```python
from build123d import *

# Parameters (mm, degrees)
SKETCH1_R            = 60
SKETCH1_R_2          = 7.9
BOSS_EXTRUDE1_DEPTH  = 8
M6_CLEARANCE_HOLE1_D = 6.6
M3_CLEARANCE_HOLE1_D = 3.6
SKETCH8_R            = 4.2
CUT_EXTRUDE1_DEPTH   = 2.7
CHAMFER1_SIZE        = 0.5


with BuildPart() as part:
    # Sketch1 → Boss-Extrude1 (new body)
    with BuildSketch(Plane.XY):
        Circle(SKETCH1_R)
        Circle(SKETCH1_R_2, mode=Mode.SUBTRACT)
    extrude(amount=BOSS_EXTRUDE1_DEPTH)

    # M6 Clearance Hole1 (through all)
    with Locations(Plane.XY.offset(8)):
        with Locations((-37.123106012, 37.123106012), (0, 52.5), (37.123106012, 37.123106012), (52.5, 0), (37.123106012, -37.123106012), (0, -52.5), (-37.123106012, -37.123106012), (-52.5, 0)):
            Hole(M6_CLEARANCE_HOLE1_D / 2)

    # M3 Clearance Hole1 (through all)
    with Locations(Plane.XY.offset(8)):
        with Locations((0, 12.5), (0, -12.5), (0, 0)):
            Hole(M3_CLEARANCE_HOLE1_D / 2)

    # Sketch8 → Cut-Extrude1 (cut)
    with BuildSketch(Plane.XY.offset(8)):
        with Locations((30, 0)):
            Circle(SKETCH8_R)
        with Locations((26.56368077, -13.941695161)):
            Circle(SKETCH8_R)
        with Locations((17.041942402, -24.689515977)):
            Circle(SKETCH8_R)
        with Locations((3.616100408, -29.781266223)):
            Circle(SKETCH8_R)
        with Locations((-10.638146611, -28.050487281)):
            Circle(SKETCH8_R)
        with Locations((-22.455322445, -19.893679747)):
            Circle(SKETCH8_R)
        with Locations((-29.128254523, -7.179469929)):
            Circle(SKETCH8_R)
        with Locations((-29.128254523, 7.179469929)):
            Circle(SKETCH8_R)
        with Locations((-22.455322445, 19.893679747)):
            Circle(SKETCH8_R)
        with Locations((-10.638146611, 28.050487281)):
            Circle(SKETCH8_R)
        with Locations((3.616100408, 29.781266223)):
            Circle(SKETCH8_R)
        with Locations((17.041942402, 24.689515977)):
            Circle(SKETCH8_R)
        with Locations((26.56368077, 13.941695161)):
            Circle(SKETCH8_R)
    extrude(amount=-CUT_EXTRUDE1_DEPTH, mode=Mode.SUBTRACT)

    # Chamfer1
    chamfer1_edges = [part.edges().sort_by_distance(p)[0] for p in [
        (25.8, 0, 5.3),
        (25.8, 0, 8),
        (-33.823106012, 37.123106012, 8),
        (-33.823106012, 37.123106012, 0),
        (-60, 0, 0),
        (-49.2, 0, 8),
        (-49.2, 0, 0),
        (-33.823106012, -37.123106012, 8),
        (-33.823106012, -37.123106012, 0),
        (3.3, -52.5, 8),
        (3.3, -52.5, 0),
        (40.423106012, -37.123106012, 8),
        (40.423106012, -37.123106012, 0),
        (55.8, 0, 8),
        (55.8, 0, 0),
        (40.423106012, 37.123106012, 8),
        (40.423106012, 37.123106012, 0),
        (-60, 0, 8),
        (-7.9, 0, 0),
        (3.3, 52.5, 8),
        (3.3, 52.5, 0),
        (-7.9, 0, 8),
        (1.8, -12.5, 8),
        (1.8, -12.5, 0),
        (1.8, 12.5, 8),
        (1.8, 12.5, 0),
        (22.36368077, -13.941695161, 5.3),
        (22.36368077, -13.941695161, 8),
        (12.841942402, -24.689515977, 5.3),
        (12.841942402, -24.689515977, 8),
        (-0.583899592, -29.781266223, 5.3),
        (-0.583899592, -29.781266223, 8),
        (-14.838146611, -28.050487281, 5.3),
        (-14.838146611, -28.050487281, 8),
        (-26.655322445, -19.893679747, 5.3),
        (-26.655322445, -19.893679747, 8),
        (-33.328254523, -7.179469929, 5.3),
        (-33.328254523, -7.179469929, 8),
        (-33.328254523, 7.179469929, 5.3),
        (-33.328254523, 7.179469929, 8),
        (-26.655322445, 19.893679747, 5.3),
        (-26.655322445, 19.893679747, 8),
        (-14.838146611, 28.050487281, 5.3),
        (-14.838146611, 28.050487281, 8),
        (-0.583899592, 29.781266223, 5.3),
        (-0.583899592, 29.781266223, 8),
        (12.841942402, 24.689515977, 5.3),
        (12.841942402, 24.689515977, 8),
        (22.36368077, 13.941695161, 5.3),
        (22.36368077, 13.941695161, 8),
    ]]
    chamfer(chamfer1_edges, length=CHAMFER1_SIZE)


solid = part.part
```
Geometry: final body of the model. Coordinates: model frame, mm. A direction names the side the tool comes from. Coordinates: 2 decimals unless noted, no trailing zeros. Answer as CSV lines item,"result". Start each with the question number.
Q1. Cut plane A-A on z = 4. Count the separate pieces of the cut face and the enclosed holes in it, then the cut area to 3 significant figures.
Q2. Pin query (flat end, axial travel): P1, Ø2, axis at x = 0, y = -12.5, coming from the +Z side; P2, Ø1.5, axis at x = -43, z = 1, coming from the -Y side; P3, Ø1.5, axis at y = 44, z = 2, coming from the +X side; P4, Ø7.5, axis at x = 52.5, y = 0, coming from the +Z side. Return the tip coordinate at first contact, or that it passes through.
Q3. Line query: line 1 (Y direction, x = 0, z = 5); line 2 (X direction, y = 2, z = 4.25); line 3 (X direction, y = 38.5, z = 3.75). Output: solid intervals per line, ascending. Write a range as from..to.
Q4. Reachability of faces 3 (the cylindrical face through (22.368, 14.126, 6.662)), 4 (the cylindrical face through (37.553, 40.395, 3.951)) from +Z, -Z, +X, -X, +Y, -Y: full face, straight path, thin tool, end or side. Return the list, or none.
Q5. Mould query, pull axis X, two halves, no side actions, for faces 1 (the cylindrical face through (55.8, 0.1, 4)), 2 (the cylindrical face through (-18.45, 21.16, 6.66)). Classes: released by +X, released by -X, zero draft, split by the parting line, or undercut.
Findings below:
1,separate pieces,"1"
1,enclosed holes,"11"
1,area,"10,800 mm2"
2,P1,"passes through"
2,P2,"stops at y = -42.6"
2,P3,"stops at x = 41.59"
2,P4,"stops at z = 7.95"
3,line 1,"y = -60..-55.8, -49.2..-14.3, -10.7..-7.9, 7.9..10.7, 14.3..49.2, 55.8..60"
3,line 2,"x = -59.97..-55.12, -49.88..-7.64, 7.64..49.88, 55.12..59.97"
3,line 3,"x = -46.02..-40.12, -34.12..34.12, 40.12..46.02"
4,face 3,"+Z"
4,face 4,"+Z, -Z"
5,face 1,"undercut"
5,face 2,"undercut"
